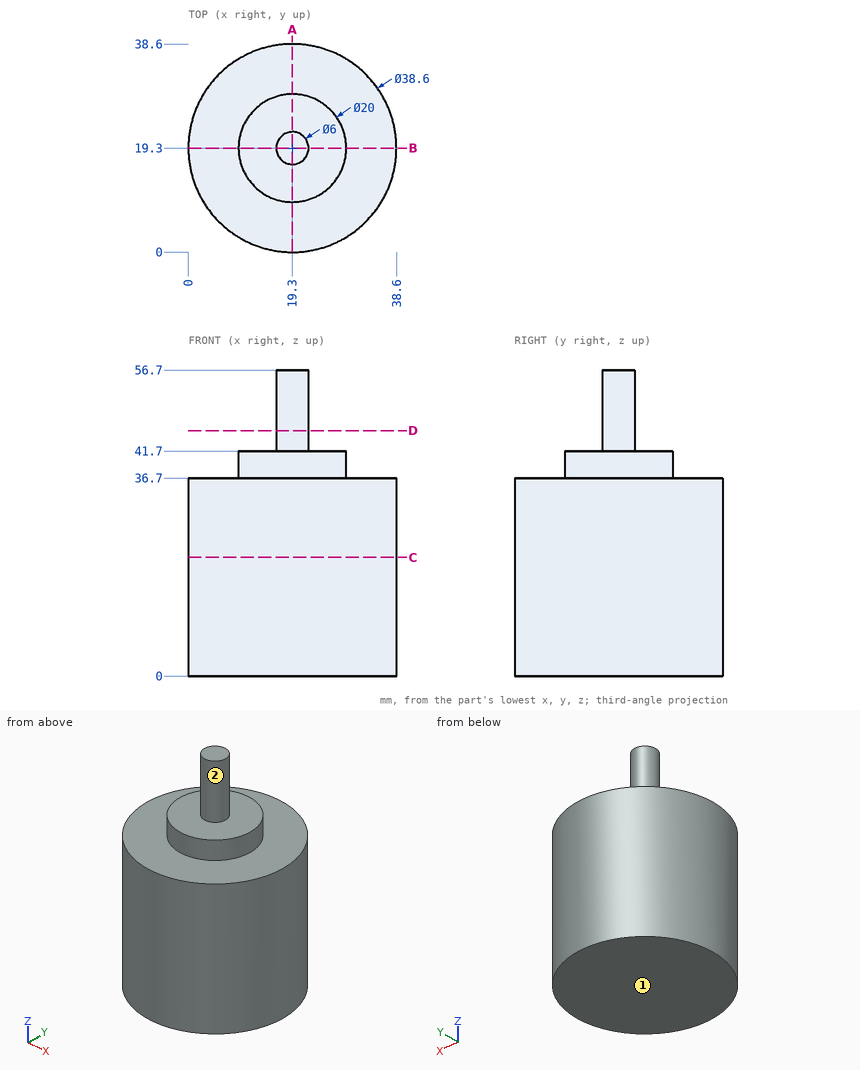
Check sheet for the drawn part. Datum: minimum x, y, z corner. Units: mm. A direction names the side the tool comes from. Coordinates: 2 decimals unless noted, no trailing zeros. Loops run counter-clockwise (first coordinate to the right, second up) from the corner with the lowest first, then second, coordinate; pieces in that order, holes last. Notation, with made-up numbers: (85, 55) -> (105, 55) arc R21 ccw to (105, 77) -> close; hole circle Ø1 at (-4, 89.5). An arc over 180 degrees is marked (long way). Answer as a JSON object with one key per item and string values. Group by question number.
Item 1: Sectioned sample at D-D on z = 45.5. Record the boundary of the cut face in (x, y), plus the area to 3 significant figures.
Item 2: Depth check by flat-ended pin: pin 1 (2 mm diameter, centred on y = 31.5, z = 19, fed in from +X); pin 2 (1 mm diameter, centred on x = 29, y = 26.5, fed in from +Z); pin 3 (6 mm diameter, centred on y = 11.5, z = 14.5, fed in from -X). Enter the tip coordinate at first touch or a pass-through.
Item 3: Sectioned sample at A-A on x = 19.3. Record the boundary of the cut face in (y, z), plus the area to 3 significant figures.
Item 4: Scan lines: probe 1 along Z at (x, y) = (11.5, 6.5); probe 2 along Z at (x, y) = (23.5, 20); probe 3 along Y at (x, z) = (19.5, 19). Record each from-to range of solid material in increasing order.
Item 5: Sectioned sample at C-C on z = 22. Record the boundary of the cut face in (x, y).
Item 6: Tool access check on the marked faces 1 and 2. Record the directions out of +Z, -Z, +X, -X, +Y, -Y that give a thin tool (end or side, any length) a straight path to the whole face; none if there is none.
Evaluation:
{
 "1": {"outline": "circle Ø6 at (19.3, 19.3)", "area": "28.3 mm²"},
 "2": {"pin 1": "stops at x = 35.02", "pin 2": "stops at z = 36.7", "pin 3": "stops at x = 0.61"},
 "3": {"outline": "(0, 0) -> (38.6, 0) -> (38.6, 36.7) -> (29.3, 36.7) -> (29.3, 41.7) -> (22.3, 41.7) -> (22.3, 56.7) -> (16.3, 56.7) -> (16.3, 41.7) -> (9.3, 41.7) -> (9.3, 36.7) -> (0, 36.7) -> close", "area": "1,610 mm²"},
 "4": {"probe 1": "z = 0 to 36.7", "probe 2": "z = 0 to 41.7", "probe 3": "y = 0 to 38.6"},
 "5": {"outline": "circle Ø38.6 at (19.3, 19.3)"},
 "6": {"face 1": "-Z, +X, -X, +Y, -Y", "face 2": "+Z"}
}
